Verification items for the finished model (mm, model axes). Face numbers are marked on the shaded views. Give positions to 0.01 mm unless a question says otherwise; leave off trailing zeros. Loops run counter-clockwise (first coordinate to the right, second up) from the corner with the lowest first, then second, coordinate; pieces in that order, holes last. Notation, with made-up numbers: (-33.75, -11.5) - (18.25, -11.5) arc R24 cw to (18.25, 12.5) - close; hole circle Ø6 at (75, -30). An arc over 180 degrees is marked (long way). One line per item, written item: value. Start each with the question number.
1. Sectioned sample at B-B (z = -1.5). Record the cut outline in (x, y).
2. Mould release check, pull along X, two halves, no side actions. Record for the marked faces 1, 2 and 3: pulls with the +X half, pulls with the -X half, needs draft (parallel to the pull), parting line crosses it, or undercut.
3. Gauge pin test, flat ends, axial feed: pin 1 (6 mm diameter, centred on x = 22.5, z = -29.5, fed in from -Y); pin 2 (1 mm diameter, centred on y = 1.5, z = -21.5, fed in from +X). Record the tip position at first contact, or that the pin passes through.
4. Scan lines: L1, parallel to X at y = -2, z = -35.5; L2, parallel to Z at x = 12, y = -3.25; L3, parallel to X at y = -2, z = 34. Record each from-to range of solid material in increasing order. Write a range as [from, to].
5. Sectioned sample at A-A (x = 0). Record the cut outline in (y, z).
from build123d import *

# Parameters (mm, degrees)
SALIENTE_EXTRUIR2_DEPTH = 3.6


with BuildPart() as part:
    # Croquis1 → Saliente-Extruir2 (new, symmetric)
    with BuildSketch(Plane(origin=(0, 0, 0), x_dir=(1, 0, 0), z_dir=(0, 1, 0))):
        with BuildLine():
            ThreePointArc((-3.841343145, 37.884615385), (0, 35), (3.841343145, 37.884615385))
            ThreePointArc((3.841343145, 37.884615385), (4.833741548, 39.729116135), (6.494598229, 41.005279406))
            ThreePointArc((6.494598229, 41.005279406), (7.679810659, 39.278343072), (8.05365555, 37.217450642))
            ThreePointArc((8.05365555, 37.217450642), (10.815594803, 33.28697807), (15.360324409, 34.843370016))
            ThreePointArc((15.360324409, 34.843370016), (16.874133455, 36.290926502), (18.848058162, 36.991396957))
            ThreePointArc((18.848058162, 36.991396957), (19.441609492, 34.98273212), (19.160306326, 32.907182521))
            ThreePointArc((19.160306326, 32.907182521), (20.57248383, 28.315594803), (25.375730098, 28.391412822))
            ThreePointArc((25.375730098, 28.391412822), (27.26276761, 29.300328129), (29.35653884, 29.35653884))
            ThreePointArc((29.35653884, 29.35653884), (29.300328129, 27.26276761), (28.391412822, 25.375730098))
            ThreePointArc((28.391412822, 25.375730098), (28.315594803, 20.57248383), (32.907182521, 19.160306326))
            ThreePointArc((32.907182521, 19.160306326), (34.98273212, 19.441609492), (36.991396957, 18.848058162))
            ThreePointArc((36.991396957, 18.848058162), (36.290926502, 16.874133455), (34.843370016, 15.360324409))
            ThreePointArc((34.843370016, 15.360324409), (33.28697807, 10.815594803), (37.217450642, 8.05365555))
            ThreePointArc((37.217450642, 8.05365555), (39.278343072, 7.679810659), (41.005279406, 6.494598229))
            ThreePointArc((41.005279406, 6.494598229), (39.729116135, 4.833741548), (37.884615385, 3.841343145))
            ThreePointArc((37.884615385, 3.841343145), (35, 0), (37.884615385, -3.841343145))
            ThreePointArc((37.884615385, -3.841343145), (39.729116135, -4.833741548), (41.005279406, -6.494598229))
            ThreePointArc((41.005279406, -6.494598229), (39.278343072, -7.679810659), (37.217450642, -8.05365555))
            ThreePointArc((37.217450642, -8.05365555), (33.28697807, -10.815594803), (34.843370016, -15.360324409))
            ThreePointArc((34.843370016, -15.360324409), (36.290926502, -16.874133455), (36.991396957, -18.848058162))
            ThreePointArc((36.991396957, -18.848058162), (34.98273212, -19.441609492), (32.907182521, -19.160306326))
            ThreePointArc((32.907182521, -19.160306326), (28.315594803, -20.57248383), (28.391412822, -25.375730098))
            ThreePointArc((28.391412822, -25.375730098), (29.300328129, -27.26276761), (29.35653884, -29.35653884))
            ThreePointArc((29.35653884, -29.35653884), (27.26276761, -29.300328129), (25.375730098, -28.391412822))
            ThreePointArc((25.375730098, -28.391412822), (20.57248383, -28.315594803), (19.160306326, -32.907182521))
            ThreePointArc((19.160306326, -32.907182521), (19.441609492, -34.98273212), (18.848058162, -36.991396957))
            ThreePointArc((18.848058162, -36.991396957), (16.874133455, -36.290926502), (15.360324409, -34.843370016))
            ThreePointArc((15.360324409, -34.843370016), (10.815594803, -33.28697807), (8.05365555, -37.217450642))
            ThreePointArc((8.05365555, -37.217450642), (7.679810659, -39.278343072), (6.494598229, -41.005279406))
            ThreePointArc((6.494598229, -41.005279406), (4.833741548, -39.729116135), (3.841343145, -37.884615385))
            ThreePointArc((3.841343145, -37.884615385), (0, -35), (-3.841343145, -37.884615385))
            ThreePointArc((-3.841343145, -37.884615385), (-4.833741548, -39.729116135), (-6.494598229, -41.005279406))
            ThreePointArc((-6.494598229, -41.005279406), (-7.679810659, -39.278343072), (-8.05365555, -37.217450642))
            ThreePointArc((-8.05365555, -37.217450642), (-10.815594803, -33.28697807), (-15.360324409, -34.843370016))
            ThreePointArc((-15.360324409, -34.843370016), (-16.874133455, -36.290926502), (-18.848058162, -36.991396957))
            ThreePointArc((-18.848058162, -36.991396957), (-19.441609492, -34.98273212), (-19.160306326, -32.907182521))
            ThreePointArc((-19.160306326, -32.907182521), (-20.57248383, -28.315594803), (-25.375730098, -28.391412822))
            ThreePointArc((-25.375730098, -28.391412822), (-27.26276761, -29.300328129), (-29.35653884, -29.35653884))
            ThreePointArc((-29.35653884, -29.35653884), (-29.300328129, -27.26276761), (-28.391412822, -25.375730098))
            ThreePointArc((-28.391412822, -25.375730098), (-28.315594803, -20.57248383), (-32.907182521, -19.160306326))
            ThreePointArc((-32.907182521, -19.160306326), (-34.98273212, -19.441609492), (-36.991396957, -18.848058162))
            ThreePointArc((-36.991396957, -18.848058162), (-36.290926502, -16.874133455), (-34.843370016, -15.360324409))
            ThreePointArc((-34.843370016, -15.360324409), (-33.28697807, -10.815594803), (-37.217450642, -8.05365555))
            ThreePointArc((-37.217450642, -8.05365555), (-39.278343072, -7.679810659), (-41.005279406, -6.494598229))
            ThreePointArc((-41.005279406, -6.494598229), (-39.729116135, -4.833741548), (-37.884615385, -3.841343145))
            ThreePointArc((-37.884615385, -3.841343145), (-35, 0), (-37.884615385, 3.841343145))
            ThreePointArc((-37.884615385, 3.841343145), (-39.729116135, 4.833741548), (-41.005279406, 6.494598229))
            ThreePointArc((-41.005279406, 6.494598229), (-39.278343072, 7.679810659), (-37.217450642, 8.05365555))
            ThreePointArc((-37.217450642, 8.05365555), (-33.28697807, 10.815594803), (-34.843370016, 15.360324409))
            ThreePointArc((-34.843370016, 15.360324409), (-36.290926502, 16.874133455), (-36.991396957, 18.848058162))
            ThreePointArc((-36.991396957, 18.848058162), (-34.98273212, 19.441609492), (-32.907182521, 19.160306326))
            ThreePointArc((-32.907182521, 19.160306326), (-28.315594803, 20.57248383), (-28.391412822, 25.375730098))
            ThreePointArc((-28.391412822, 25.375730098), (-29.300328129, 27.26276761), (-29.35653884, 29.35653884))
            ThreePointArc((-29.35653884, 29.35653884), (-27.26276761, 29.300328129), (-25.375730098, 28.391412822))
            ThreePointArc((-25.375730098, 28.391412822), (-20.57248383, 28.315594803), (-19.160306326, 32.907182521))
            ThreePointArc((-19.160306326, 32.907182521), (-19.441609492, 34.98273212), (-18.848058162, 36.991396957))
            ThreePointArc((-18.848058162, 36.991396957), (-16.874133455, 36.290926502), (-15.360324409, 34.843370016))
            ThreePointArc((-15.360324409, 34.843370016), (-10.815594803, 33.28697807), (-8.05365555, 37.217450642))
            ThreePointArc((-8.05365555, 37.217450642), (-7.679810659, 39.278343072), (-6.494598229, 41.005279406))
            ThreePointArc((-6.494598229, 41.005279406), (-4.833741548, 39.729116135), (-3.841343145, 37.884615385))
        make_face()
    extrude(amount=SALIENTE_EXTRUIR2_DEPTH, both=True)


solid = part.part
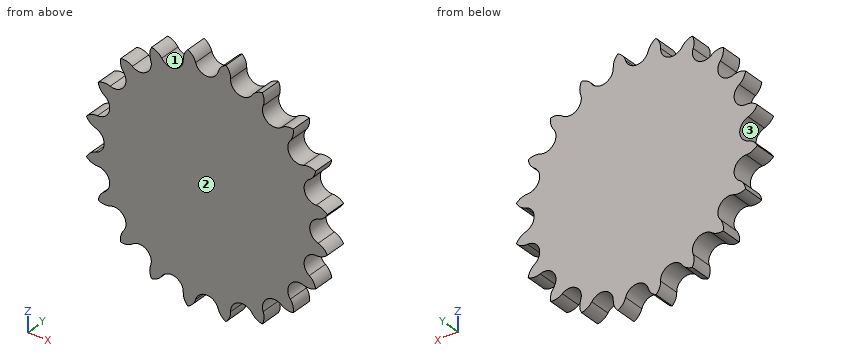
Results are:
1. outline: (-35.29, -3.6) - (35.29, -3.6) - (35.29, 3.6) - (-35.29, 3.6) - close
2. face 1: undercut
2. face 2: needs draft
2. face 3: pulls with the -X half
3. pin 1: stops at y = -3.6
3. pin 2: stops at x = 28.04
4. L1: x = [-19.37, -15.89], [-8.38, -1.94], [1.94, 8.38], [15.89, 19.37]
4. L2: z = [-33.09, 33.09]
4. L3: x = [-19.42, -14.59], [-9.51, 9.51], [14.59, 19.42]
5. outline: (-3.6, -35) - (3.6, -35) - (3.6, 35) - (-3.6, 35) - close
